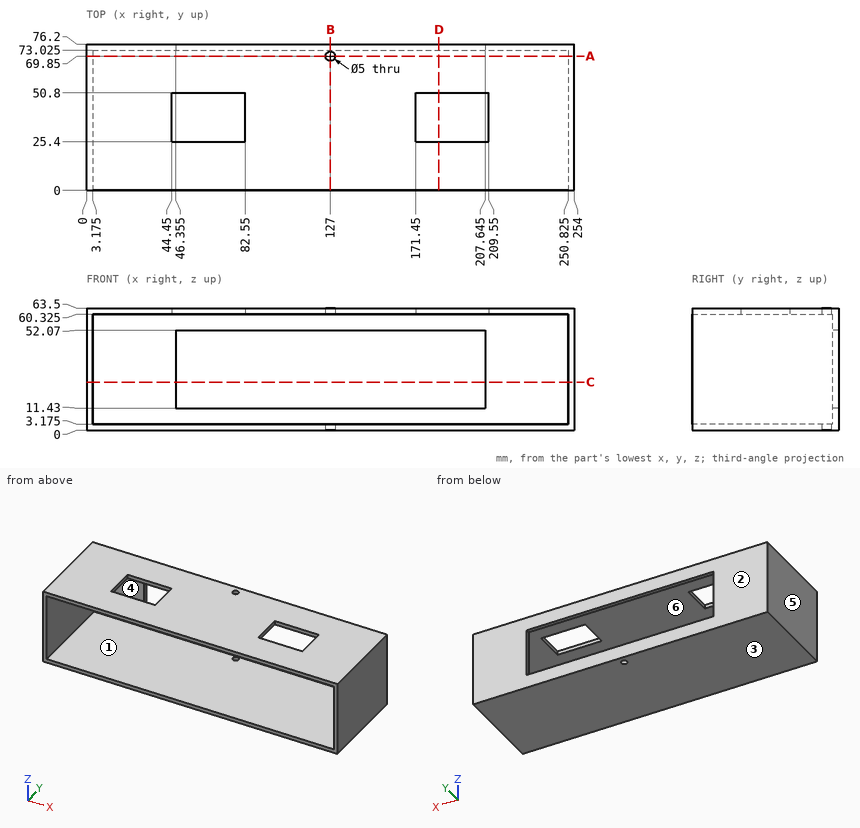
Geometry check sheet. Reference: drawing and pictorial views, mm from the part's lowest x, y, z. A direction names the side the tool comes from. Coordinates: 2 decimals unless noted, no trailing zeros. Order: outer loops, then holes, each group sorted by start corner. A loop starts at its lowest first (then second) coordinate and runs counter-clockwise, first axis right, second up. Notation, with made-up numbers: M 77,-39 L 124,-39 A37 cw 124,-1 Z; hole C 75.25,76.5 d1. An arc over 180 degrees is marked long. Write each question's results on one line, items separated by ' | '. Start each with the question number.
1. Go/stop test with flat-tipped pins: P1, Ø12, axis at x = 179, z = 11, coming from the -Y side (3 decimals); P2, Ø2.5, axis at y = 75.5, z = 22, coming from the -X side. Record where each tip stops, or that it passes through.
2. Cross-section at C-C on z = 25. Record the cut outline in (x, y) (3 decimals).
3. Cross-section at A-A on y = 69.85. Record the cut outline in (x, z) (3 decimals), and give its area (3 significant figures).
4. Cross-section at B-B on x = 127. Record the cut outline in (y, z) (3 decimals), and give its area (3 significant figures).
5. Access from +Z, -Z, +X, -X, +Y, -Y to the whole of each face (thin tool, end or side, straight path). Record for the marked faces 1 and 2.
6. Mould release check, pull along X, two halves, no side actions. Record for the marked faces 3, 4, 5 and 6: +X half, -X half, draft (parallel to the pull), parting line (faces both ways), or undercut.
7. Material ranges on probe 1 along X at (y, z) = (62.5, 7) (3 decimals); probe 2 along Y at (x, z) = (127, 61); probe 3 along Z at (x, y) = (184.5, 71) (3 decimals), recorded low to high.
8. Cross-section at D-D on x = 183.5. Record the cut outline in (y, z) (3 decimals), and give its area (3 significant figures).
Checks:
1) P1: stops at y = 73.025 | P2: stops at x = 0
2) outline: M 0,0 L 3.175,0 L 3.175,73.025 L 46.355,73.025 L 46.355,76.2 L 0,76.2 Z; M 207.645,73.025 L 250.825,73.025 L 250.825,0 L 254,0 L 254,76.2 L 207.645,76.2 Z
3) outline: M 0,0 L 124.5,0 L 124.5,3.175 L 3.175,3.175 L 3.175,60.325 L 124.5,60.325 L 124.5,63.5 L 0,63.5 Z; M 129.5,0 L 254,0 L 254,63.5 L 129.5,63.5 L 129.5,60.325 L 250.825,60.325 L 250.825,3.175 L 129.5,3.175 Z | area: 1,940 mm²
4) outline: M 0,0 L 67.35,0 L 67.35,3.175 L 0,3.175 Z; M 0,60.325 L 67.35,60.325 L 67.35,63.5 L 0,63.5 Z; M 72.35,0 L 76.2,0 L 76.2,11.43 L 73.025,11.43 L 73.025,3.175 L 72.35,3.175 Z; M 72.35,60.325 L 73.025,60.325 L 73.025,52.07 L 76.2,52.07 L 76.2,63.5 L 72.35,63.5 Z | area: 505 mm²
5) face 1: -Y | face 2: +Z, -Z, +X, -X, +Y
6) face 3: draft | face 4: undercut | face 5: -X half | face 6: undercut
7) probe 1: x = 0 to 3.175, 250.825 to 254 | probe 2: y = 0 to 67.35, 72.35 to 76.2 | probe 3: z = 0 to 3.175, 60.325 to 63.5
8) outline: M 0,0 L 76.2,0 L 76.2,11.43 L 73.025,11.43 L 73.025,3.175 L 0,3.175 Z; M 0,60.325 L 25.4,60.325 L 25.4,63.5 L 0,63.5 Z; M 50.8,60.325 L 73.025,60.325 L 73.025,52.07 L 76.2,52.07 L 76.2,63.5 L 50.8,63.5 Z | area: 456 mm²
